Autodesk Inventor part; units mm, degrees
ref_plane "YZ Plane" through (0, 0, 0) normal (1, 0, 0) x (0, 1, 0)
ref_plane "XZ Plane" through (0, 0, 0) normal (0, 1, 0) x (-1, 0, 0)
ref_plane "XY Plane" through (0, 0, 0) normal (0, 0, 1) x (1, 0, 0)
sketch "Sketch1" plane through (0, 0, 0) normal (0, 1, 0) x (-1, 0, 0)
  line L0 (51.3, 38.5) -> (51.3, -38.5)
  line L1 (51.3, -38.5) -> (38.5, -38.5)
  line L2 (38.5, -38.5) -> (38.5, -51.3)
  line L3 (38.5, -51.3) -> (-38.5, -51.3)
  line L4 (-38.5, -51.3) -> (-38.5, -38.5)
  line L5 (-38.5, -38.5) -> (-51.3, -38.5)
  line L6 (-51.3, -38.5) -> (-51.3, 38.5)
  line L7 (-51.3, 38.5) -> (-38.5, 38.5)
  line L8 (-38.5, 38.5) -> (-38.5, 51.3)
  line L9 (-38.5, 51.3) -> (38.5, 51.3)
  line L10 (38.5, 51.3) -> (38.5, 38.5)
  line L11 (38.5, 38.5) -> (51.3, 38.5)
  circle A0 centre (0, 0) radius 5
  dimension "d0" = 77
  dimension "d1" = 12.8
  dimension "d2" = 12.8
  dimension "d3" = 77
  dimension "d4" = 12.8
  dimension "d5" = 12.8
  dimension "d6" = 77
  dimension "d7" = 12.8
  dimension "d8" = 12.8
  dimension "d9" = 77
  dimension "d10" = 12.8
  dimension "d11" = 12.8
  dimension "d12" = 38.5
  dimension "d13" = 51.3
  dimension "d14" = 10
extrude "Extrusion1" add sketch "Sketch1" along normal blind 11.5
sketch "Sketch2" plane through (38.5, 0, 51.3) normal (1, 0, 0) x (0, 0, -1)
  circle A0 centre (6.4, 9) radius 1.65
  line L0 (0, 0) -> (0, 11.5)
  line L1 (0, 11.5) -> (12.8, 11.5)
  point P0 (51.3, 0)
  dimension "d17" = 3.3
  dimension "d18" = 6.4
  dimension "d19" = 2.5
hole "Hole1" at (38.5, 9, 44.9) direction (-1, 0, 0) diameter 3.3 depth 10 tip angle 118
thread "Thread1"
sketch "Sketch3" plane through (-38.5, 0, 51.3) normal (0, 0, 1) x (1, 0, 0)
  circle A0 centre (68, 9) radius 0.5
  line L0 (0, 11.5) -> (77, 11.5)
  line L1 (77, 0) -> (77, 11.5)
  point P0 (38.5, 0)
  dimension "d29" = 1
  dimension "d30" = 2.5
  dimension "d31" = 9
hole "Hole2" at (29.5, 9, 51.3) direction (0, 0, -1) diameter 2 depth 5 tip angle 118
sketch "Sketch4" plane through (-38.5, 0, 38.5) normal (-1, 0, 0) x (0, 0, 1)
  circle A0 centre (6.4, 9) radius 1.65
  line L0 (0, 11.5) -> (12.8, 11.5)
  line L1 (12.8, 0) -> (12.8, 11.5)
  point P0 (-38.5, 0)
  dimension "d39" = 3.3
  dimension "d40" = 2.5
  dimension "d41" = 6.4
hole "Hole3" at (-38.5, 9, 44.9) direction (1, 0, 0) diameter 3.3 depth 10 tip angle 118
thread "Thread2"
sketch "Sketch5" plane through (-38.5, 0, 51.3) normal (0, 0, 1) x (1, 0, 0)
  circle A0 centre (9, 9) radius 1
  line L0 (0, 0) -> (0, 11.5)
  line L1 (0, 11.5) -> (77, 11.5)
  point P0 (38.5, 0)
  dimension "d51" = 2
  dimension "d52" = 9
  dimension "d53" = 2.5
hole "Hole4" at (-29.5, 9, 51.3) direction (0, 0, -1) diameter 2 depth 5 tip angle 118
sketch "Sketch6" plane through (38.5, 0, -38.5) normal (1, 0, 0) x (0, 0, -1)
  circle A0 centre (6.4, 9) radius 1.65
  line L0 (0, 11.5) -> (12.8, 11.5)
  line L1 (12.8, 0) -> (12.8, 11.5)
  point P0 (-38.5, 0)
  dimension "d61" = 3.3
  dimension "d62" = 2.5
  dimension "d63" = 6.4
hole "Hole5" at (38.5, 9, -44.9) direction (-1, 0, 0) diameter 3.3 depth 10 tip angle 118
thread "Thread3"
sketch "Sketch7" plane through (38.5, 0, -51.3) normal (0, 0, -1) x (-1, 0, 0)
  circle A0 centre (9, 9) radius 1
  line L0 (0, 0) -> (0, 11.5)
  line L1 (0, 11.5) -> (77, 11.5)
  point P0 (38.5, 0)
  dimension "d73" = 2
  dimension "d74" = 9
  dimension "d75" = 2.5
hole "Hole6" at (29.5, 9, -51.3) direction (0, 0, 1) diameter 2 depth 5 tip angle 118
sketch "Sketch8" plane through (-38.5, 0, -51.3) normal (-1, 0, 0) x (0, 0, 1)
  circle A0 centre (6.4, 9) radius 1.65
  line L0 (0, 11.5) -> (12.8, 11.5)
  line L1 (0, 0) -> (0, 11.5)
  point P0 (51.3, 0)
  dimension "d83" = 3.3
  dimension "d84" = 2.5
  dimension "d85" = 6.4
hole "Hole7" at (-38.5, 9, -44.9) direction (1, 0, 0) diameter 3.3 depth 10 tip angle 118
thread "Thread4"
sketch "Sketch9" plane through (38.5, 0, -51.3) normal (0, 0, -1) x (-1, 0, 0)
  circle A0 centre (68, 9) radius 1
  line L0 (0, 11.5) -> (77, 11.5)
  line L1 (77, 0) -> (77, 11.5)
  point P0 (38.5, 0)
  dimension "d95" = 2
  dimension "d96" = 2.5
  dimension "d97" = 9
hole "Hole8" at (-29.5, 9, -51.3) direction (0, 0, 1) diameter 2 depth 5 tip angle 118
properties part number "PEEKplate"
Here's how the part is built. I have some questions about the finished solid (model axes, mm). A direction names the side the tool comes from. Give positions to 0.01 mm unless a question says otherwise; leave off trailing zeros. Order: outer loops, then holes, each group sorted by start corner. A loop starts at its lowest first (then second) coordinate and runs counter-clockwise, first axis right, second up. Notation, with made-up numbers: M 72.25,37.25 L 108.25,37.25 A23 cw 108.25,54.25 Z; hole C 73.25,74.25 d10. An arc over 180 degrees is marked long. Answer as a JSON object with one key per item and string values. Group by question number.
1) Suppose I cut it at C-C, the plane y = 4.5. Write out the boundary of the cut face in (x, z), plus the area to 3 significant figures.
2) I'm going to push flat-ended pins straight in: pin 1 Ø6 at (y, z) = (6.5, -42) entering from -X; pin 2 Ø2 at (y, z) = (9, 44.9) entering from +X; pin 3 Ø3.5 at (x, y) = (43.5, 4.5) entering from +Z. Where does each tip first touch, or does it pass through?
3) Suppose I cut it at B-B, the plane x = 0. Write out the boundary of the cut face in (y, z).
4) Please list where these lines run through material, in increasing order: L1, parallel to X at y = 9, z = -48.3; L2, parallel to Z at x = 32.5, y = 9; L3, parallel to Z at x = 0, y = 10.25. Write a range as [from, to].
5) We'd pull the mould along X, two halves only. Please class faces 1 (the flat face through (-45, 6, 38.5)), 2 (the cylindrical face through (1.08, 5.67, 4.88)), 3 (the conical face through (-27.681, 9.013, -45.186)), 4 (the conical face through (27.681, 9.013, -44.614)): pulls with the +X half, pulls with the -X half, needs draft (parallel to the pull), parting line crosses it, or undercut.
6) On a 3-axis mill with a long thin cutter (end or side, diameter ignored), from which of +Z, -Z, +X, -X, +Y, -Y can I reach the whole of each face in a straight line? I mean faces 5 (the flat face through (38.5, 6, 45)), 6 (the cylindrical face through (33.43, 8.93, -43.25)), 7 (the cylindrical face through (-33.43, 9.632, -43.376)), 8 (the flat face through (-38.5, 6, 45)), 9 (the flat face through (-38.5, 6, -45)). Say none if no direction works.
7) Suppose I cut it at A-A, the plane z = 0. Write out the boundary of the cut face in (x, y).
Results found:
{
 "1": {"outline": "M -51.3,-38.5 L -38.5,-38.5 L -38.5,-51.3 L 38.5,-51.3 L 38.5,-38.5 L 51.3,-38.5 L 51.3,38.5 L 38.5,38.5 L 38.5,51.3 L -38.5,51.3 L -38.5,38.5 L -51.3,38.5 Z; hole C 0,0 d10", "area": "9,790 mm²"},
 "2": {"pin 1": "x = -38.5", "pin 2": "x = 28.11", "pin 3": "z = 38.5"},
 "3": {"outline": "M 0,-51.3 L 11.5,-51.3 L 11.5,-5 L 0,-5 Z; M 0,5 L 11.5,5 L 11.5,51.3 L 0,51.3 Z"},
 "4": {"L1": "[-38.5, -30.5], [-28.5, 28.5], [30.5, 38.5]", "L2": "[-51.3, -46.55], [-43.25, 43.25], [46.55, 51.3]", "L3": "[-51.3, -5], [5, 51.3]"},
 "5": {"face 1": "needs draft", "face 2": "undercut", "face 3": "pulls with the -X half", "face 4": "pulls with the +X half"},
 "6": {"face 5": "+Z, +X, +Y, -Y", "face 6": "+X", "face 7": "-X", "face 8": "+Z, -X, +Y, -Y", "face 9": "-Z, -X, +Y, -Y"},
 "7": {"outline": "M -51.3,0 L -5,0 L -5,11.5 L -51.3,11.5 Z; M 5,0 L 51.3,0 L 51.3,11.5 L 5,11.5 Z"}
}
